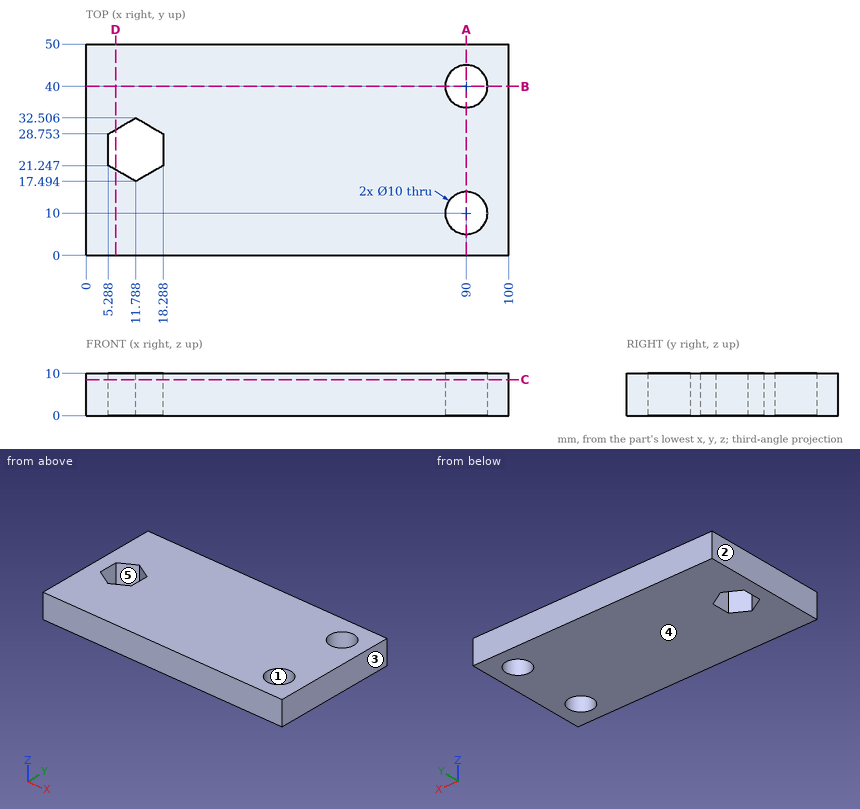
Design review of the part shown in the three views and the two pictorial views. Dimensions are in mm from the part's minimum x, y and z. A direction names the side the tool comes from. Round coordinates to 2 decimals unless told otherwise and drop trailing zeros. Loops run counter-clockwise (first coordinate to the right, second up) from the corner with the lowest first, then second, coordinate; pieces in that order, holes last. Notation, with made-up numbers: (70, 76) -> (106, 76) arc R13 ccw to (106, 86) -> close; hole circle Ø5 at (42.5, -10). An arc over 180 degrees is marked (long way). Return JSON: item names as keys, results as strings.
(1) For the marked faces 4 and 5, list the 3-axis set-ups (+Z, -Z, +X, -X, +Y, -Y) from which the entire face can be reached by the end or side of a thin tool; tool diameter is ignored.
Solved:
{"face 4": "-Z, +X, -X, +Y, -Y", "face 5": "+Z, -Z"}
(2) Add section A-A on x = 90. Write out the cut boundary in (y, z).
Solved:
{"outline": "(0, 0) -> (5, 0) -> (5, 10) -> (0, 10) -> close; (15, 0) -> (35, 0) -> (35, 10) -> (15, 10) -> close; (45, 0) -> (50, 0) -> (50, 10) -> (45, 10) -> close"}
(3) For line 1 (Y direction, x = 90, z = 4); line 2 (X direction, y = 25, z = 4.25); line 3 (Y direction, x = 89, z = 5.75), list the stretches that pass through material, from the lowest coordinate up.
Solved:
{"line 1": "0 to 5, 15 to 35, 45 to 50", "line 2": "0 to 5.29, 18.29 to 100", "line 3": "0 to 5.1, 14.9 to 35.1, 44.9 to 50"}
(4) Add section C-C on z = 8.5. Write out the cut boundary in (x, y) (1 decimal).
Solved:
{"outline": "(0, 0) -> (100, 0) -> (100, 50) -> (0, 50) -> close; hole (5.3, 21.2) -> (11.8, 17.5) -> (18.3, 21.2) -> (18.3, 28.8) -> (11.8, 32.5) -> (5.3, 28.8) -> close; hole circle Ø10 at (90, 10); hole circle Ø10 at (90, 40)"}
(5) Add section B-B on y = 40. Write out the cut boundary in (x, z).
Solved:
{"outline": "(0, 0) -> (85, 0) -> (85, 10) -> (0, 10) -> close; (95, 0) -> (100, 0) -> (100, 10) -> (95, 10) -> close"}
(6) The part is to be moulded in two halves that separate along X. For the marked faces 1, 2 and 3, say which applies: released by +X, released by -X, zero draft, split by the parting line, or undercut.
Solved:
{"face 1": "undercut", "face 2": "released by -X", "face 3": "released by +X"}
(7) Add section D-D on x = 7. Write out the cut boundary in (y, z), plus the area to 3 significant figures.
Solved:
{"outline": "(0, 0) -> (20.26, 0) -> (20.26, 10) -> (0, 10) -> close; (29.74, 0) -> (50, 0) -> (50, 10) -> (29.74, 10) -> close", "area": "405 mm2"}
